Input: dimensioned drawing with shaded views. Units: mm. Origin: part minimum x, y, z. Coordinates: 2 decimals unless noted, no trailing zeros. Order: outer loops, then holes, each group sorted by start corner. A loop starts at its lowest first (then second) coordinate and runs counter-clockwise, first axis right, second up. Notation, with made-up numbers: (-20.75, 20) -> (2.25, 20) arc R11 cw to (2.25, 29) -> close; hole circle Ø5 at (-22, 88). An arc over 180 degrees is marked (long way). Answer in a Markdown table with one row per item. Add a question column.
1) Section query C-C on z = 0.8. Return the cut outline in (x, y) (3 decimals), then the cut area to 3 significant figures.
2) Contact query for a flat-ended pin moving along its axis: P1, Ø2.5, axis at x = 65.555, y = 15, coming from the +Z side. Output: stop coordinate, or through.
3) Ray query, line 1 (X direction, y = 15, z = 1.5) (3 decimals); line 2 (X direction, y = 12, z = 0.15); line 3 (Y direction, x = 51, z = 0.75). Return the intervals inside material, ascending. Write a range as from..to.
4) Section query B-B on y = 19. Return the cut outline in (x, z).
5) Section query D-D on y = 15. Return the cut outline in (x, z) (3 decimals), then the cut area to 3 significant figures.
6) Section query A-A on x = 34. Return the cut outline in (y, z).
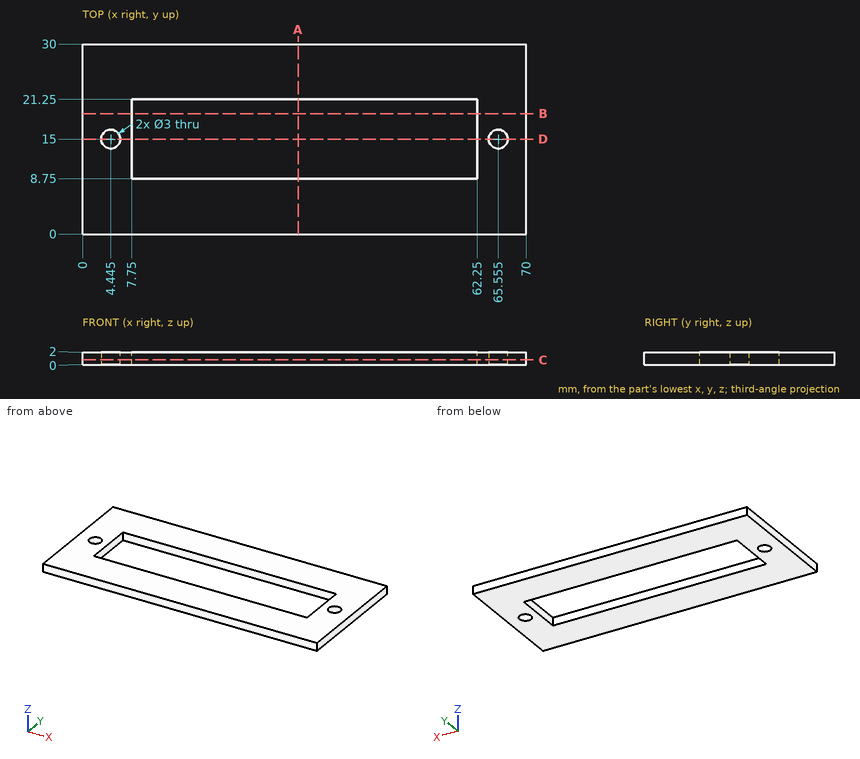
Result:
| question | item | result |
|---|---|---|
| 1 | outline | (0, 0) -> (70, 0) -> (70, 30) -> (0, 30) -> close; hole circle Ø3 at (4.445, 15); hole (7.75, 8.75) -> (62.25, 8.75) -> (62.25, 21.25) -> (7.75, 21.25) -> close; hole circle Ø3 at (65.555, 15) |
| 1 | area | 1,400 mm2 |
| 2 | P1 | through |
| 3 | line 1 | 0..2.945, 5.945..7.75, 62.25..64.055, 67.055..70 |
| 3 | line 2 | 0..7.75, 62.25..70 |
| 3 | line 3 | 0..8.75, 21.25..30 |
| 4 | outline | (0, 0) -> (7.75, 0) -> (7.75, 2) -> (0, 2) -> close; (62.25, 0) -> (70, 0) -> (70, 2) -> (62.25, 2) -> close |
| 5 | outline | (0, 0) -> (2.945, 0) -> (2.945, 2) -> (0, 2) -> close; (5.945, 0) -> (7.75, 0) -> (7.75, 2) -> (5.945, 2) -> close; (62.25, 0) -> (64.055, 0) -> (64.055, 2) -> (62.25, 2) -> close; (67.055, 0) -> (70, 0) -> (70, 2) -> (67.055, 2) -> close |
| 5 | area | 19.0 mm2 |
| 6 | outline | (0, 0) -> (8.75, 0) -> (8.75, 2) -> (0, 2) -> close; (21.25, 0) -> (30, 0) -> (30, 2) -> (21.25, 2) -> close |
